Part print with two shaded views. Sizes in mm from the minimum x, y, z corner. A direction names the side the tool comes from. Coordinates: 2 decimals unless noted, no trailing zeros. Order: outer loops, then holes, each group sorted by start corner. A loop starts at its lowest first (then second) coordinate and runs counter-clockwise, first axis right, second up.
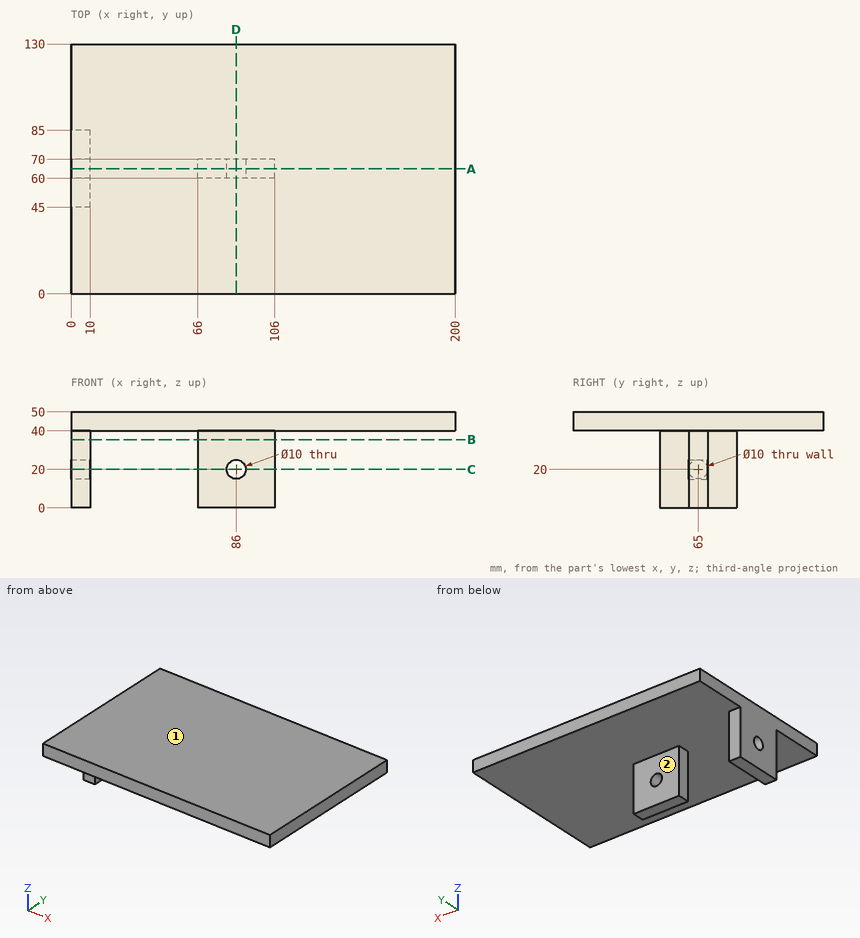
Q1. Cut at D-D on x = 86. Write the cut outline in (y, z).
Results list:
outline: (0, 40) - (60, 40) - (60, 25) - (70, 25) - (70, 40) - (130, 40) - (130, 50) - (0, 50) - close; (60, 0) - (70, 0) - (70, 15) - (60, 15) - close
Q2. Cut at C-C on z = 20. Write the cut outline in (x, y).
Results list:
outline: (0, 45) - (10, 45) - (10, 60) - (0, 60) - close; (0, 70) - (10, 70) - (10, 85) - (0, 85) - close; (66, 60) - (81, 60) - (81, 70) - (66, 70) - close; (91, 60) - (106, 60) - (106, 70) - (91, 70) - close
Q3. Which spindle directions (+Z, -Z, +X, -X, +Y, -Y) get a long thin tool onto all of the face, cutting with end or side? Do the marked faces 1 and 2. Say none if no direction does.
Results list:
face 1: +Z, +X, -X, +Y, -Y
face 2: -Z, +X, +Y
Q4. Cut at B-B on z = 35.5. Write the cut outline in (x, y), and give its area (3 significant figures).
Results list:
outline: (0, 45) - (10, 45) - (10, 85) - (0, 85) - close; (66, 60) - (106, 60) - (106, 70) - (66, 70) - close
area: 800 mm2
Q5. Wall check: line 1 along X through (y, z) = (67.5, 20); line 2 along Z through (x, y) = (86, 65); line 3 along Y through (x, z) = (4, 20). Give the ranges that are in metal, low to high.
Results list:
line 1: x = 66 to 81, 91 to 106
line 2: z = 0 to 15, 25 to 50
line 3: y = 45 to 60, 70 to 85
Q6. Pin check, flat tips, straight feed: pin 1 Ø9 at (x, z) = (86, 20) entering from -Y; pin 2 Ø20 at (x, z) = (89, 28) entering from +Y; pin 3 Ø20 at (x, z) = (87, 25.5) entering from -Y; pin 4 Ø4 at (x, y) = (38.5, 115.5) entering from -Z. Stop position of each tip, or through.
Results list:
pin 1: passes through
pin 2: stops at y = 70
pin 3: stops at y = 60
pin 4: stops at z = 40
Q7. Cut at A-A on y = 65. Write the cut outline in (x, z).
Results list:
outline: (0, 0) - (10, 0) - (10, 15) - (0, 15) - close; (0, 25) - (10, 25) - (10, 40) - (66, 40) - (66, 0) - (106, 0) - (106, 40) - (200, 40) - (200, 50) - (0, 50) - close; hole circle Ø10 at (86, 20)
